For this review, take the finished solid that the model builds, in its own axes (mm). Face numbers are marked on the shaded views. A direction names the side the tool comes from. Give positions to 0.01 mm unless a question says otherwise; leave off trailing zeros. Order: outer loops, then holes, each group sorted by start corner. A loop starts at its lowest first (then second) coordinate and runs counter-clockwise, first axis right, second up.
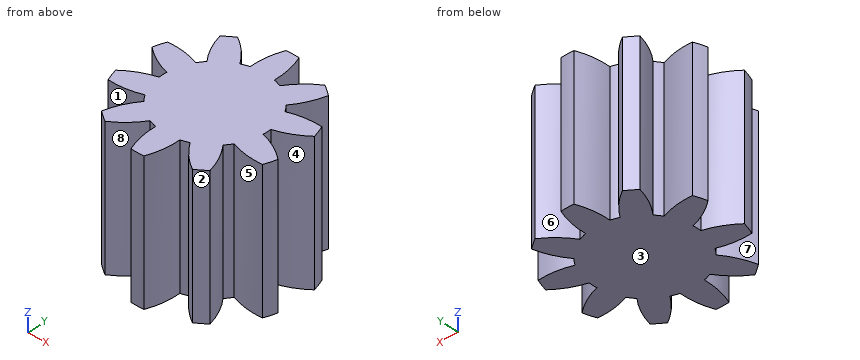
Autodesk Inventor part; units mm, degrees
ref_plane "Work Plane2" through (0, 0, 10) normal (0, 0, 1) x (1, 0, 0)
ref_plane "Work Plane8" through (0, 0, 0) normal (0.9510565, 0.309017, 0) x (0, 0, 1)
ref_plane "Work Plane9" through (0, 0, 0) normal (1, 0, 0) x (0, 1, 0)
sketch "Sketch1" plane through (0, 0, 0) normal (0, 0, 1) x (1, 0, 0)
  circle A0 centre (0, 0) radius 12
  dimension "d0" = 24
extrude "Extrusion1" add sketch "Sketch1" along normal blind 20
ref_plane "Work Plane2" through (0, 0, 10) normal (0, 0, 1) x (1, 0, 0)
sketch "Sketch2" plane through (0, 0, 0) normal (0, 0, -1) x (-1, 0, 0)
  circle A0 centre (0, 0) radius 12
  circle A1 centre (0, 0) radius 10
  dimension "d3" = 20
surface extrude "Средний диаметр" sketch "Sketch2" against normal through all shown no curves A1
ref_plane "Work Plane8" through (0, 0, 0) normal (0.9510565, 0.309017, 0) x (0, 0, 1)
ref_plane "Work Plane9" through (0, 0, 0) normal (1, 0, 0) x (0, 1, 0)
spur gear teeth "Цилиндрическое зубчатое зацепление" teeth 10 pitch diameter 20 tip diameter 24 root diameter 15 face width 20 start plane through (0, 0, 0) normal (0, 0, -1) x (-1, 0, 0)
equation "\"d0\" = da_da"
equation "\"d1\" = da_b"
equation "\"d3\" = da_dw"
properties part number "Цилиндрическое зубчатое зацепление1" material "Steel"
1) We need section A-A on y = -8.5. Give the boundary of the cut face in (x, z).
Answer sheet:
outline: (-7.62, 0) - (-4.12, 0) - (-4.12, 20) - (-7.62, 20) - close; (-1.74, 0) - (1.74, 0) - (1.74, 20) - (-1.74, 20) - close; (4.12, 0) - (7.62, 0) - (7.62, 20) - (4.12, 20) - close
2) We need section B-B on x = 9.5. Give the boundary of the cut face in (y, z).
Answer sheet:
outline: (-4.6, 0) - (-1.37, 0) - (-1.37, 20) - (-4.6, 20) - close; (1.37, 0) - (4.6, 0) - (4.6, 20) - (1.37, 20) - close
3) To check wall thickness, follow line 1 (X direction, y = -9, z = 14.5); line 2 (X direction, y = -8.75, z = 11); line 3 (Y direction, x = 6.5, z = 18). State the ranges of each line that lie inside material, in increasing order.
Answer sheet:
line 1: x = -7.76 to -4.64, -1.7 to 1.7, 4.64 to 7.76
line 2: x = -7.7 to -4.37, -1.72 to 1.72, 4.37 to 7.7
line 3: y = -10.09 to -6.01, -3.96 to 3.96, 6.01 to 10.09
4) Clearance check with flat-ended pins moving along their axes: pin 1 (2 mm diameter, centred on y = 9.5, z = 7, fed in from +X); pin 2 (2 mm diameter, centred on x = 5.5, z = 17, fed in from +Y); pin 3 (1 mm diameter, centred on x = 3, z = 9, fed in from -Y). State where each tip first meets the part, or that it passes through.
Answer sheet:
pin 1: stops at x = 7.79
pin 2: stops at y = 10.23
pin 3: stops at y = -7.79
5) Draft analysis for pull direction X (two halves, no side actions). For the marked faces 1, 2 and 3, state which applies: +X half, -X half, draft (parallel to the pull), parting line (faces both ways), or undercut.
Answer sheet:
face 1: undercut
face 2: +X half
face 3: draft
6) Tool access review of the marked faces 4, 5, 6, 7 and 8: name each direction out of +Z, -Z, +X, -X, +Y, -Y from which nothing blocks a thin tool from reaching the whole face with its end or side.
Answer sheet:
face 4: +Z, -Z, +X
face 5: +Z, -Z
face 6: +Z, -Z, +Y
face 7: +Z, -Z, -X
face 8: +Z, -Z, -Y
7) We need section D-D on x = -4.25. Give the boundary of the cut face in (y, z), then the cut area to 3 significant figures.
Answer sheet:
outline: (-8.63, 0) - (8.63, 0) - (8.63, 20) - (-8.63, 20) - close
area: 345 mm2
8) We need section C-C on y = 8. Give the boundary of the cut face in (x, z), then the cut area to 3 significant figures.
Answer sheet:
outline: (-7.45, 0) - (-3.67, 0) - (-3.67, 20) - (-7.45, 20) - close; (-1.76, 0) - (1.76, 0) - (1.76, 20) - (-1.76, 20) - close; (3.67, 0) - (7.45, 0) - (7.45, 20) - (3.67, 20) - close
area: 222 mm2
